For this review, take the finished solid that the model builds, in its own axes (mm). A direction names the side the tool comes from. Give positions to 0.01 mm unless a question says otherwise; leave off trailing zeros. Write each loop counter-clockwise with the first axis right and the second up, starting at its lowest first coordinate (ties: lowest second). Pieces come first, ordered by that corner, then holes. Notation, with made-up numbers: M 73.25,-10.75 L 105.25,-10.75 A18 ccw 105.25,2.25 Z; hole C 35,3 d1. An arc over 180 degrees is marked long. Write item = value, one per line.
```python
from build123d import *
from build123d.topology import SkipClean

# Parameters (mm, degrees)
BOSS_EXTRUDE1_DEPTH = 2
SKETCH2_R           = 1.6
BOSS_EXTRUDE3_DEPTH = 6
BOSS_EXTRUDE4_START = 4
SKETCH5_R           = 16
SKETCH5_R_2         = 7.5
BOSS_EXTRUDE4_DEPTH = 4
BOSS_EXTRUDE7_START = 1
SKETCH6_R           = 16
BOSS_EXTRUDE7_DEPTH = 1
BOSS_EXTRUDE8_START = -5
SKETCH7_R           = 1.6
BOSS_EXTRUDE8_DEPTH = 5


with BuildPart() as part:
    # Sketch1 → Boss-Extrude1 (new body)
    # profile 1 of 2: a face of its own
    with BuildSketch(Plane.XY):
        with BuildLine():
            ThreePointArc((15.491933385, 4), (9.797958971, 12.649110641), (0, 16))
            ThreePointArc((0, 16), (-9.797958971, 12.649110641), (-15.491933385, 4))
            ThreePointArc((-15.491933385, 4), (-16, 0), (-15.491933385, -4))
            ThreePointArc((-15.491933385, -4), (0, -16), (15.491933385, -4))
            ThreePointArc((15.491933385, -4), (15.87247514, -2.01606868), (16, 0))
            ThreePointArc((16, 0), (15.87247514, 2.01606868), (15.491933385, 4))
        make_face()
        with BuildLine():
            ThreePointArc((7.5, 0), (-5.303300859, -5.303300859), (0, 7.5))
            ThreePointArc((0, 7.5), (5.303300859, 5.303300859), (7.5, 0))
        make_face(mode=Mode.SUBTRACT)
    # profile 2 of 2: a face of its own
    with BuildSketch(Plane.XY):
        with BuildLine():
            ThreePointArc((15.491933385, 4), (9.797958971, 12.649110641), (0, 16))
            ThreePointArc((0, 16), (-9.797958971, 12.649110641), (-15.491933385, 4))
            ThreePointArc((-15.491933385, 4), (-16, 0), (-15.491933385, -4))
            ThreePointArc((-15.491933385, -4), (0, -16), (15.491933385, -4))
            ThreePointArc((15.491933385, -4), (15.87247514, -2.01606868), (16, 0))
            ThreePointArc((16, 0), (15.87247514, 2.01606868), (15.491933385, 4))
        make_face()
        with BuildLine():
            ThreePointArc((7.5, 0), (-5.303300859, -5.303300859), (0, 7.5))
            ThreePointArc((0, 7.5), (5.303300859, 5.303300859), (7.5, 0))
        make_face(mode=Mode.SUBTRACT)
    extrude(amount=BOSS_EXTRUDE1_DEPTH)

    # Sketch2 → Boss-Extrude3 (add)
    # profile 1 of 2: a face of its own
    with BuildSketch(Plane.XY):
        with BuildLine():
            Line((-20, -4), (-15.491933385, -4))
            ThreePointArc((-15.491933385, -4), (-16, 0), (-15.491933385, 4))
            Line((-15.491933385, 4), (-20, 4))
            ThreePointArc((-20, 4), (-24, 0), (-20, -4))
        make_face()
        with Locations((-20, 0)):
            Circle(SKETCH2_R, mode=Mode.SUBTRACT)
    # profile 2 of 2: a face of its own
    with BuildSketch(Plane.XY):
        with BuildLine():
            Line((15.491933385, -4), (20, -4))
            ThreePointArc((20, -4), (24, 0), (20, 4))
            Line((20, 4), (15.491933385, 4))
            ThreePointArc((15.491933385, 4), (15.87247514, 2.01606868), (16, 0))
            ThreePointArc((16, 0), (15.87247514, -2.01606868), (15.491933385, -4))
        make_face()
        with Locations((20, 0)):
            Circle(SKETCH2_R, mode=Mode.SUBTRACT)
    extrude(amount=BOSS_EXTRUDE3_DEPTH)

    # Sketch5 → Boss-Extrude4 (add)
    with SkipClean():  # the faces are left unmerged after this step: merging them gives an invalid solid
        with BuildSketch(Plane(origin=(0, 0, 0), x_dir=(-1, 0, 0), z_dir=(0, 0, -1)).offset(BOSS_EXTRUDE4_START)):
            Circle(SKETCH5_R)
            Circle(SKETCH5_R_2, mode=Mode.SUBTRACT)
        extrude(amount=-BOSS_EXTRUDE4_DEPTH)

    # Sketch6 → Boss-Extrude7 (add)
    with SkipClean():  # the faces are left unmerged after this step: merging them gives an invalid solid
        with BuildSketch(Plane(origin=(0, 0, -4), x_dir=(-1, 0, 0), z_dir=(0, 0, -1)).offset(BOSS_EXTRUDE7_START)):
            Circle(SKETCH6_R)
        extrude(amount=-BOSS_EXTRUDE7_DEPTH)

    # Sketch7 → Boss-Extrude8 (add)
    # profile 1 of 2: a face of its own
    with SkipClean():  # the faces are left unmerged after this step: merging them gives an invalid solid
        with BuildSketch(Plane.XY.offset(BOSS_EXTRUDE8_START)):
            with BuildLine():
                Line((15.491933385, -4), (20, -4))
                ThreePointArc((20, -4), (24, 0), (20, 4))
                Line((20, 4), (15.491933385, 4))
                ThreePointArc((15.491933385, 4), (15.87247514, 2.01606868), (16, 0))
                ThreePointArc((16, 0), (15.87247514, -2.01606868), (15.491933385, -4))
            make_face()
            with Locations((20, 0)):
                Circle(SKETCH7_R, mode=Mode.SUBTRACT)
        # profile 2 of 2: a face of its own
        with BuildSketch(Plane.XY.offset(BOSS_EXTRUDE8_START)):
            with BuildLine():
                Line((-20, -4), (-15.491933385, -4))
                ThreePointArc((-15.491933385, -4), (-16, 0), (-15.491933385, 4))
                Line((-15.491933385, 4), (-20, 4))
                ThreePointArc((-20, 4), (-24, 0), (-20, -4))
            make_face()
            with Locations((-20, 0)):
                Circle(SKETCH7_R, mode=Mode.SUBTRACT)
        extrude(amount=BOSS_EXTRUDE8_DEPTH)


solid = part.part
```
1. For line 1 along Y through (x, z) = (20, 1.3); line 2 along Z through (x, y) = (13, -7.5); line 3 along Y through (x, z) = (4, 0), list the stretches that pass through material, from the lowest coordinate up. Write a range as from..to.
Responses:
line_1 = -4..-1.6, 1.6..4
line_2 = -5..2
line_3 = -15.49..-6.34, 6.34..15.49
2. We need section C-C, the plane x = -3. Write out the cut boundary in (y, z), then the cut area to 3 significant figures.
Responses:
outline = M -15.72,-5 L 15.72,-5 L 15.72,2 L 6.87,2 L 6.87,-4 L -6.87,-4 L -6.87,2 L -15.72,2 Z
area = 138 mm2
3. Insertion check: P1, Ø4, axis at y = 5.5, z = 3, coming from the -X side; P2, Ø9.5, axis at x = -0.5, y = -4.5, coming from the +Z side; P3, Ø2.5, axis at x = -17, z = -3, coming from the -Y side; P4, Ø1.9, axis at x = -20, y = 0, coming from the -Z side. Each pin has a flat end and moves straight along its axis. Give the tip position at first contact, or say it passes through.
Responses:
P1 = -21.94
P2 = 2
P3 = -4
P4 = through
4. Machinability: for faces 1 (the face through (-18, 0, 6)), 2 (the face through (0, 0, -4)), which of the approach directions +Z, -Z, +X, -X, +Y, -Y give a long, thin tool a straight path to every point of the face, cutting with its end or side? Answer none if there is none.
Responses:
face_1 = +Z, +X, -X, +Y, -Y
face_2 = +Z
5. The part is to be moulded in two halves that separate along Y. For faces 3 (the face through (-16, 0, 4)), 4 (the face through (18, -4, 0)), 5 (the face through (20, 2, 6)), say which applies: +Y half, -Y half, draft (parallel to the pull), parting line (faces both ways), or undercut.
Responses:
face_3 = undercut
face_4 = -Y half
face_5 = draft
6. We need section B-B, the plane z = 1.25. Write out the cut boundary in (x, y), then the cut area to 3 significant figures.
Responses:
outline = M -20,-4 L -15.49,-4 A16 ccw 15.49,-4 L 20,-4 A4 ccw 20,4 L 15.49,4 A16 ccw -15.49,4 L -20,4 A4 ccw Z; hole C -20,0 d3.2; hole C 0,0 d15; hole C 20,0 d3.2
area = 728 mm2
7. We need section A-A, the plane y = -1. Write out the cut boundary in (x, z), then the cut area to 3 significant figures.
Responses:
outline = M -23.87,-5 L -21.25,-5 L -21.25,6 L -23.87,6 Z; M -18.75,-5 L 18.75,-5 L 18.75,6 L 15.97,6 L 15.97,2 L 7.43,2 L 7.43,-4 L -7.43,-4 L -7.43,2 L -15.97,2 L -15.97,6 L -18.75,6 Z; M 21.25,-5 L 23.87,-5 L 23.87,6 L 21.25,6 Z
area = 253 mm2
8. We need section D-D, the plane y = -11. Write out the cut boundary in (x, z), then the cut area to 3 significant figures.
Responses:
outline = M -11.62,-5 L 11.62,-5 L 11.62,2 L -11.62,2 Z
area = 163 mm2
